Here's how the part is built. I have some questions about the finished solid (model axes, mm). Face numbers are marked on the shaded views. A direction names the side the tool comes from. Give positions to 0.01 mm unless a question says otherwise; leave off trailing zeros. Order: outer loops, then holes, each group sorted by start corner. A loop starts at its lowest first (then second) coordinate and runs counter-clockwise, first axis right, second up. Notation, with made-up numbers: M -2,43.5 L 52,43.5 A22 cw 52,63.5 Z; hole C -9,85.25 d2. An arc over 180 degrees is marked long. Use one line per item in the form item = value.
from build123d import *

# Parameters (mm, degrees)
SKETCH2_R           = 16.5
BOSS_EXTRUDE1_DEPTH = 1
SKETCH3_R           = 12
BOSS_EXTRUDE2_DEPTH = 8
BOSS_EXTRUDE3_START = 2
SKETCH4_R           = 12
BOSS_EXTRUDE3_DEPTH = 2
SKETCH5_R           = 6
CUT_EXTRUDE1_DEPTH  = 6
SKETCH6_R           = 8
CUT_EXTRUDE2_DEPTH  = 1


with BuildPart() as part:
    # Sketch2 → Boss-Extrude1 (new, symmetric)
    with BuildSketch(Plane(origin=(0, 0, 0), x_dir=(1, 0, 0), z_dir=(0, 1, 0))):
        with Locations(Location((0, 0, 0), (0, 0, 270))):
            Circle(SKETCH2_R)
    extrude(amount=BOSS_EXTRUDE1_DEPTH, both=True)

    # Sketch3 → Boss-Extrude2 (add)
    with BuildSketch(Plane.XZ.offset(1)):
        with Locations(Location((0, 0, 0), (0, 0, 270))):
            Circle(SKETCH3_R)
    extrude(amount=BOSS_EXTRUDE2_DEPTH)

    # Sketch4 → Boss-Extrude3 (add)
    with BuildSketch(Plane(origin=(0, 1, 0), x_dir=(1, 0, 0), z_dir=(0, 1, 0)).offset(BOSS_EXTRUDE3_START)):
        with Locations(Location((0, 0, 0), (0, 0, 90))):
            Circle(SKETCH4_R)
    extrude(amount=-BOSS_EXTRUDE3_DEPTH)

    # Sketch5 → Cut-Extrude1 (cut)
    with BuildSketch(Plane(origin=(0, 3, 0), x_dir=(1, 0, 0), z_dir=(0, 1, 0))):
        with Locations(Location((0, 0, 0), (0, 0, 270))):
            Circle(SKETCH5_R)
    extrude(amount=-CUT_EXTRUDE1_DEPTH, mode=Mode.SUBTRACT)

    # Sketch6 → Cut-Extrude2 (cut)
    with BuildSketch(Plane(origin=(0, 3, 0), x_dir=(1, 0, 0), z_dir=(0, 1, 0))):
        with Locations(Location((0, 0, 0), (0, 0, 270))):
            Circle(SKETCH6_R)
    extrude(amount=-CUT_EXTRUDE2_DEPTH, mode=Mode.SUBTRACT)


solid = part.part
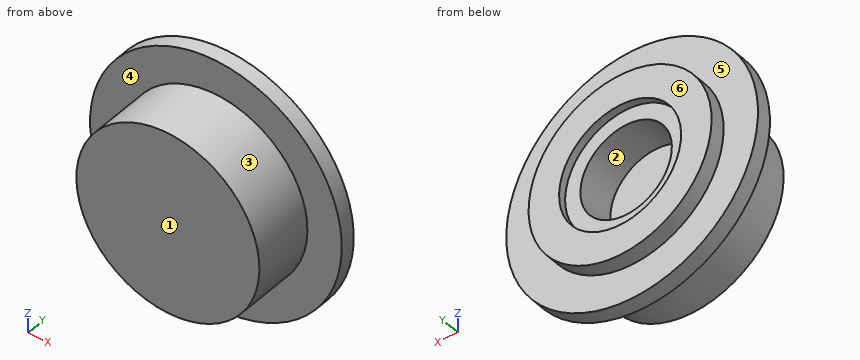
Q1. I need wall thicknesses on L1, parallel to X at y = 2.45, z = 0; L2, parallel to X at y = -1.35, z = 0; L3, parallel to Y at x = 14, z = -2.5. Which ranges of each line are inside material? Lowest first, please.
Found:
L1 = -12 to -8, 8 to 12
L2 = -12 to -6, 6 to 12
L3 = -1 to 1
Q2. I'm going to push flat-ended pins straight in: pin 1 Ø3.5 at (x, z) = (3, 1.5) entering from +Y; pin 2 Ø6 at (x, z) = (-11.5, 13) entering from +Y; pin 3 Ø1.5 at (y, z) = (-2, -10.5) entering from -X; pin 4 Ø10 at (x, z) = (-6.5, 0) entering from +Y. Where does each tip first touch, or does it pass through?
Found:
pin_1 = -3
pin_2 = 1
pin_3 = -7
pin_4 = 3
Q3. I want a section at D-D on z = 7. Write out the boundary of the cut face in (x, y).
Found:
outline = M -14.94,-1 L -9.75,-1 L -9.75,-9 L 9.75,-9 L 9.75,-1 L 14.94,-1 L 14.94,1 L 9.75,1 L 9.75,3 L 3.87,3 L 3.87,2 L -3.87,2 L -3.87,3 L -9.75,3 L -9.75,1 L -14.94,1 Z
Q4. Thinking about a two-plate mould opening in X: for the marked faces 1, 2 and 3, which applies, +X half, -X half, draft (parallel to the pull), parting line (faces both ways), or undercut?
Found:
face_1 = draft
face_2 = undercut
face_3 = parting line
Q5. I want a section at B-B on z = 0. Write out the boundary of the cut face in (x, y), then the cut area to 3 significant figures.
Found:
outline = M -16.5,-1 L -12,-1 L -12,-9 L 12,-9 L 12,-1 L 16.5,-1 L 16.5,1 L 12,1 L 12,3 L 8,3 L 8,2 L 6,2 L 6,-3 L -6,-3 L -6,2 L -8,2 L -8,3 L -12,3 L -12,1 L -16.5,1 Z
area = 230 mm²
Q6. I want a section at C-C on y = -6. Write out the boundary of the cut face in (x, z), then the cut area to 3 significant figures.
Found:
outline = C 0,0 d24
area = 452 mm²
Q7. I want a section at A-A on x = 0. Write out the boundary of the cut face in (y, z), then the cut area to 3 significant figures.
Found:
outline = M -9,-12 L -1,-12 L -1,-16.5 L 1,-16.5 L 1,-12 L 3,-12 L 3,-8 L 2,-8 L 2,-6 L -3,-6 L -3,6 L 2,6 L 2,8 L 3,8 L 3,12 L 1,12 L 1,16.5 L -1,16.5 L -1,12 L -9,12 Z
area = 230 mm²
Q8. On a 3-axis mill with a long thin cutter (end or side, diameter ignored), from which of +Z, -Z, +X, -X, +Y, -Y can I reach the whole of each face in a straight line? I mean the marked faces 4, 5 and 6. Say none if no direction works.
Found:
face_4 = -Y
face_5 = +Y
face_6 = +Z, -Z, +X, -X, +Y
